```python
from build123d import *

# Parameters (mm, degrees)
SKETCH1_R           = 3.175
BOSS_EXTRUDE1_DEPTH = 3.175


with BuildPart() as part:
    # Sketch1 → Boss-Extrude1 (new body)
    with BuildSketch(Plane(origin=(0, 0, 0), x_dir=(1, 0, 0), z_dir=(0, 1, 0))):
        with BuildLine():
            Line((0, 161.169349013), (114.3, 161.169349013))
            Line((114.3, 161.169349013), (114.3, 148.469349013))
            Line((114.3, 148.469349013), (120.65, 148.469349013))
            Line((120.65, 148.469349013), (120.65, 142.119349013))
            ThreePointArc((120.65, 142.119349013), (122.509871939, 137.629220953), (127, 135.769349013))
            Line((127, 135.769349013), (133.35, 135.769349013))
            ThreePointArc((133.35, 135.769349013), (142.875, 126.244349013), (133.35, 116.719349013))
            Line((133.35, 116.719349013), (127, 116.719349013))
            ThreePointArc((127, 116.719349013), (122.509871939, 114.859477074), (120.65, 110.369349013))
            Line((120.65, 110.369349013), (120.65, 84.969349013))
            Line((120.65, 84.969349013), (114.3, 84.969349013))
            Line((114.3, 84.969349013), (114.3, 72.269349013))
            Line((114.3, 72.269349013), (120.65, 72.269349013))
            Line((120.65, 72.269349013), (120.65, 46.869349013))
            ThreePointArc((120.65, 46.869349013), (122.509871939, 42.379220953), (127, 40.519349013))
            Line((127, 40.519349013), (133.35, 40.519349013))
            ThreePointArc((133.35, 40.519349013), (142.875, 30.994349013), (133.35, 21.469349013))
            Line((133.35, 21.469349013), (127, 21.469349013))
            ThreePointArc((127, 21.469349013), (122.509871939, 19.609477074), (120.65, 15.119349013))
            Line((120.65, 15.119349013), (120.65, 8.769349013))
            Line((120.65, 8.769349013), (114.3, 8.769349013))
            Line((114.3, 8.769349013), (114.3, -3.930650987))
            Line((114.3, -3.930650987), (0, -3.930650987))
            Line((0, -3.930650987), (0, 8.769349013))
            Line((0, 8.769349013), (-6.35, 8.769349013))
            Line((-6.35, 8.769349013), (-6.35, 15.119349013))
            ThreePointArc((-6.35, 15.119349013), (-8.209871939, 19.609477074), (-12.7, 21.469349013))
            Line((-12.7, 21.469349013), (-19.05, 21.469349013))
            ThreePointArc((-19.05, 21.469349013), (-28.575, 30.994349013), (-19.05, 40.519349013))
            Line((-19.05, 40.519349013), (-12.7, 40.519349013))
            ThreePointArc((-12.7, 40.519349013), (-8.209871939, 42.379220953), (-6.35, 46.869349013))
            Line((-6.35, 46.869349013), (-6.35, 72.269349013))
            Line((-6.35, 72.269349013), (0, 72.269349013))
            Line((0, 72.269349013), (0, 84.969349013))
            Line((0, 84.969349013), (-6.35, 84.969349013))
            Line((-6.35, 84.969349013), (-6.35, 110.369349013))
            ThreePointArc((-6.35, 110.369349013), (-8.209871939, 114.859477074), (-12.7, 116.719349013))
            Line((-12.7, 116.719349013), (-19.05, 116.719349013))
            ThreePointArc((-19.05, 116.719349013), (-28.575, 126.244349013), (-19.05, 135.769349013))
            Line((-19.05, 135.769349013), (-12.7, 135.769349013))
            ThreePointArc((-12.7, 135.769349013), (-8.209871939, 137.629220953), (-6.35, 142.119349013))
            Line((-6.35, 142.119349013), (-6.35, 148.469349013))
            Line((-6.35, 148.469349013), (0, 148.469349013))
            Line((0, 148.469349013), (0, 161.169349013))
        make_face()
        with Locations(Location((-19.05, 126.244349013, 0), (0, 0, 270))):
            Circle(SKETCH1_R, mode=Mode.SUBTRACT)
        with Locations(Location((-19.05, 30.994349013, 0), (0, 0, 270))):
            Circle(SKETCH1_R, mode=Mode.SUBTRACT)
        with Locations(Location((133.35, 30.994349013, 0), (0, 0, 270))):
            Circle(SKETCH1_R, mode=Mode.SUBTRACT)
        with Locations(Location((133.35, 126.244349013, 0), (0, 0, 270))):
            Circle(SKETCH1_R, mode=Mode.SUBTRACT)
        with BuildLine():
            Line((107.95, 126.185693187), (107.95, 31.05300484))
            ThreePointArc((107.95, 31.05300484), (103.340232575, 24.946116059), (96.203829737, 27.705790103))
            Line((96.203829737, 27.705790103), (66.698688048, 75.272134277))
            ThreePointArc((66.698688048, 75.272134277), (65.744858311, 78.619349013), (66.698688048, 81.96656375))
            Line((66.698688048, 81.96656375), (96.203829737, 129.532907923))
            ThreePointArc((96.203829737, 129.532907923), (103.340232575, 132.292581968), (107.95, 126.185693187))
        make_face(mode=Mode.SUBTRACT)
        with BuildLine():
            Line((81.593842457, 8.769349013), (32.706157543, 8.769349013))
            ThreePointArc((32.706157543, 8.769349013), (27.157404819, 12.031656799), (27.30998728, 18.46656375))
            Line((27.30998728, 18.46656375), (51.753829737, 57.873397836))
            ThreePointArc((51.753829737, 57.873397836), (57.15, 60.876183099), (62.546170263, 57.873397836))
            Line((62.546170263, 57.873397836), (86.99001272, 18.46656375))
            ThreePointArc((86.99001272, 18.46656375), (87.142595181, 12.031656799), (81.593842457, 8.769349013))
        make_face(mode=Mode.SUBTRACT)
        with BuildLine():
            Line((6.35, 126.185693187), (6.35, 31.05300484))
            ThreePointArc((6.35, 31.05300484), (10.959767425, 24.946116059), (18.096170263, 27.705790103))
            Line((18.096170263, 27.705790103), (47.601311952, 75.272134277))
            ThreePointArc((47.601311952, 75.272134277), (48.555141689, 78.619349013), (47.601311952, 81.96656375))
            Line((47.601311952, 81.96656375), (18.096170263, 129.532907923))
            ThreePointArc((18.096170263, 129.532907923), (10.959767425, 132.292581968), (6.35, 126.185693187))
        make_face(mode=Mode.SUBTRACT)
        with BuildLine():
            Line((86.99001272, 138.772134277), (62.546170263, 99.36530019))
            ThreePointArc((62.546170263, 99.36530019), (57.15, 96.362514927), (51.753829737, 99.36530019))
            Line((51.753829737, 99.36530019), (27.30998728, 138.772134277))
            ThreePointArc((27.30998728, 138.772134277), (27.157404819, 145.207041228), (32.706157543, 148.469349013))
            Line((32.706157543, 148.469349013), (81.593842457, 148.469349013))
            ThreePointArc((81.593842457, 148.469349013), (87.142595181, 145.207041228), (86.99001272, 138.772134277))
        make_face(mode=Mode.SUBTRACT)
    extrude(amount=BOSS_EXTRUDE1_DEPTH)


solid = part.part
```
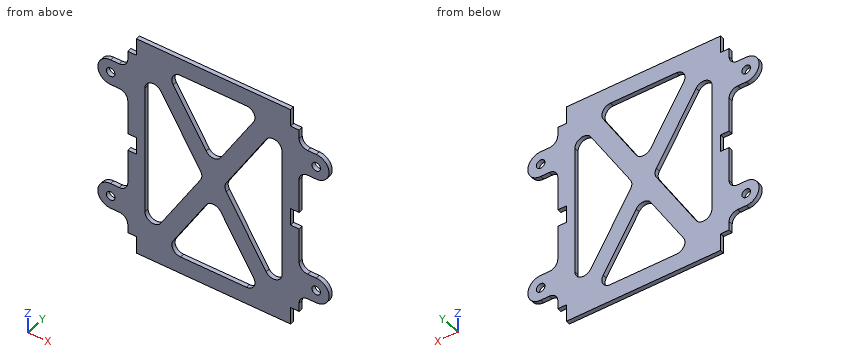
Work out the finished part from the listing and answer in its coordinate system (mm). Round coordinates to 2 decimals unless told otherwise and drop trailing zeros. Write each loop counter-clockwise with the first axis right and the second up, starting at its lowest first coordinate (ties: lowest second). Pieces come first, ordered by that corner, then holes. Notation, with made-up numbers: (27, -4.75) -> (58, -4.75) arc R35 cw to (58, 31.25) -> close; hole circle Ø6 at (-4.75, 48). An arc over 180 degrees is marked (long way). Write each question's results on one line, items separated by ' | '.
Q1. Section B-B, the plane z = -105 is taken. Write down the section's boundary in (x, y) (3 decimals), then the cut area to 3 significant figures.
Data:
outline: (-6.35, 0) -> (6.35, 0) -> (6.35, 3.175) -> (-6.35, 3.175) -> close; (33.314, 0) -> (48.259, 0) -> (48.259, 3.175) -> (33.314, 3.175) -> close; (66.041, 0) -> (80.986, 0) -> (80.986, 3.175) -> (66.041, 3.175) -> close; (107.95, 0) -> (120.65, 0) -> (120.65, 3.175) -> (107.95, 3.175) -> close | area: 176 mm^2
Q2. Flat-ended cylindrical pins translate along their axes: P1, Ø1.6, axis at y = 1.5, z = -13, coming from the +X side; P2, Ø1.6, axis at y = 2, z = 0, coming from the -X side; P3, Ø1.6, axis at x = 129.5, y = 1.5, coming from the -Z side. Find the tip coordinate at first contact, or state that the pin passes through.
Data:
P1: x = 120.65 | P2: x = 0 | P3: z = -135.77
Q3. Straight lines are drawn through the part: line 1 along Z through (x, y) = (133.35, 1.2); line 2 along X through (y, z) = (2.4, -123); line 3 along Z through (x, y) = (64.5, 0.9). For each, find the intervals that lie inside material, in ascending order. Write a range as [from, to].
Data:
line 1: [-135.77, -129.42], [-123.07, -116.72], [-40.52, -34.17], [-27.82, -21.47] | line 2: [-28.01, 6.35], [22.15, 37.09], [77.21, 92.15], [107.95, 142.31] | line 3: [-161.17, -148.47], [-102.52, -54.72], [-8.77, 3.93]
Q4. Section D-D, the plane y = 1.15 is taken. Give the number of separate pieces and of enclosed holes in the cut face, then the cut area to 3 significant figures.
Data:
separate pieces: 1 | enclosed holes: 8 | area: 12,300 mm^2
Q5. Section A-A, the plane x = 9 is taken. Write down the section's boundary in (y, z) (3 decimals).
Data:
outline: (0, -161.169) -> (3.175, -161.169) -> (3.175, -131.346) -> (0, -131.346) -> close; (0, -25.892) -> (3.175, -25.892) -> (3.175, 3.931) -> (0, 3.931) -> close
Q6. Section C-C, the plane z = -87.5 is taken. Write down the section's boundary in (x, y) (3 decimals), then the cut area to 3 significant figures.
Data:
outline: (-6.35, 0) -> (6.35, 0) -> (6.35, 3.175) -> (-6.35, 3.175) -> close; (44.169, 0) -> (70.131, 0) -> (70.131, 3.175) -> (44.169, 3.175) -> close; (107.95, 0) -> (120.65, 0) -> (120.65, 3.175) -> (107.95, 3.175) -> close | area: 163 mm^2
